Check sheet for the modelled part. Datum: model origin and axes. Units: mm. Face numbers are marked on the shaded views. A direction names the side the tool comes from. Give positions to 0.01 mm unless a question says otherwise; leave off trailing zeros. Write each loop counter-clockwise with the first axis right and the second up, starting at its lowest first coordinate (ties: lowest second). Pieces come first, ordered by that corner, then holes. Notation, with made-up numbers: M 17.5,-37 L 33.5,-37 A19 cw 33.5,-2 Z; hole C 3,17 d6. An arc over 180 degrees is marked long. Use CSV: the item, a comma, the result in double quotes. Start each with the question number.
1. Depth check by flat-ended pin: P1, Ø0.6, axis at y = 0, z = 0.5, coming from the -X side; P2, Ø1, axis at x = -1.5, y = -1, coming from the -Z side. Enter the tip coordinate at first touch or a pass-through.
2. Access from +Z, -Z, +X, -X, +Y, -Y to the whole of each face (thin tool, end or side, straight path). Record for the marked faces 5, 6, 7, 8 and 9.
3. Mould release check, pull along X, two halves, no side actions. Record for the marked faces 1, 2, 3 and 4: +X half, -X half, draft (parallel to the pull), parting line (faces both ways), or undercut.
4. Cross-section at A-A, the plane z = 1.4. Enter the section's corners in (x, y) (3 decimals), and give its area (3 significant figures).
5. Scan lines: line 1 (X direction, y = 1.5, z = 1.35); line 2 (Z direction, x = -3, y = 1); line 3 (Z direction, x = -1.25, y = 1.5). Record each from-to range of solid material in increasing order.
6. Cross-section at D-D, the plane z = 2.5. Enter the section's corners in (x, y).
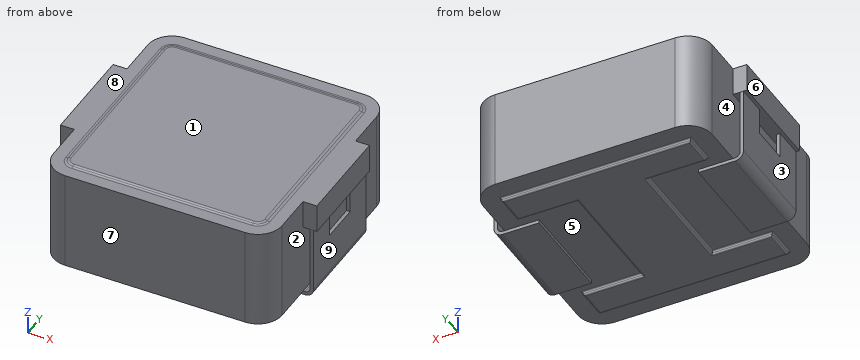
from build123d import *

# Parameters (mm, degrees)
SKETCH1_W            = 6.6
SKETCH1_H            = 6.6
BOSS_EXTRUDE1_DEPTH  = 2.9
SKETCH6_W            = 7.4
SKETCH6_H            = 2.9
BOSS_EXTRUDE5_DEPTH  = 0.85
FILLET1_R            = 0.7
SKETCH2_W            = 0.9
SKETCH2_H            = 2.1
CUT_EXTRUDE1_DEPTH   = 0.05
SKETCH3_W            = 1.3
SKETCH3_H            = 2.89
BOSS_EXTRUDE2_DEPTH  = 0.15
SKETCH4_W            = 0.3
SKETCH4_H            = 2.89
BOSS_EXTRUDE3_DEPTH  = 2
FILLET2_R            = 0.25
BOSS_EXTRUDE4_DEPTH  = 0.1
FILLET3_R            = 0.05
FILLET4_R            = 0.05
SKETCH8_W            = 0.2
SKETCH8_H            = 2.89
CUT_EXTRUDE2_DEPTH   = 2.05
FILLET5_R            = 0.15
SKETCH9_W            = 0.75
SKETCH9_H            = 1.15
CUT_EXTRUDE3_DEPTH   = 0.1
FILLET2_OF_MIRROR2_R = 0.25
FILLET5_OF_MIRROR2_R = 0.15
SKETCH10_W           = 10
SKETCH10_H           = 10
CUT_EXTRUDE4_DEPTH   = 0.03
FILLET6_R            = 0.2
FILLET7_R            = 0.2


# Some blends are built 0.0001 mm under size
with BuildPart() as part:
    # Sketch1 → Boss-Extrude1 (new body)
    with BuildSketch(Plane.XY):
        Rectangle(SKETCH1_W, SKETCH1_H)
    extrude(amount=BOSS_EXTRUDE1_DEPTH)

    # Sketch6 → Boss-Extrude5 (add)
    with BuildSketch(Plane.XY.offset(2.9)):
        Rectangle(SKETCH6_W, SKETCH6_H)
    extrude(amount=-BOSS_EXTRUDE5_DEPTH)

    # Fillet1
    fillet1_edges = [part.edges().sort_by_distance(p)[0] for p in [
        (3.3, -3.3, 1.45),
        (-3.3, -3.3, 1.45),
        (-3.3, 3.3, 1.45),
        (3.3, 3.3, 1.45),
    ]]
    fillet(fillet1_edges, radius=FILLET1_R)

    # Sketch2 → Cut-Extrude1 (cut)
    with BuildSketch(Plane(origin=(0, 0, 0), x_dir=(-1, 0, 0), z_dir=(0, 0, -1))):
        with Locations((2.85, 0)):
            Rectangle(SKETCH2_W, SKETCH2_H)
        with Locations((-2.85, 0)):
            Rectangle(SKETCH2_W, SKETCH2_H)
    extrude(amount=-CUT_EXTRUDE1_DEPTH, mode=Mode.SUBTRACT)

    # Sketch3 → Boss-Extrude2 (add)
    with BuildSketch(Plane(origin=(0, 0, 0.05), x_dir=(-1, 0, 0), z_dir=(0, 0, -1))):
        with Locations((2.95, 0)):
            Rectangle(SKETCH3_W, SKETCH3_H)
    boss_extrude2 = extrude(amount=BOSS_EXTRUDE2_DEPTH)

    # Sketch4 → Boss-Extrude3 (add)
    with BuildSketch(Plane.XY.offset(0.05)):
        with Locations((-3.45, 0)):
            Rectangle(SKETCH4_W, SKETCH4_H)
    boss_extrude3 = extrude(amount=BOSS_EXTRUDE3_DEPTH)

    # Fillet2
    fillet2_edges = [part.edges().sort_by_distance(p)[0] for p in [
        (-3.6, 0, -0.1),
    ]]
    fillet(fillet2_edges, radius=FILLET2_R)

    # Sketch5 → Boss-Extrude4 (add)
    with BuildSketch(Plane(origin=(0, 0, 0), x_dir=(-1, 0, 0), z_dir=(0, 0, -1))):
        Polygon((2.725, -2.7), (-2.725, -2.7), (-2.725, -1.8), (-1, -1.8), (-1, 1.8), (-2.725, 1.8), (-2.725, 2.7), (2.725, 2.7), (2.725, 1.8), (1, 1.8), (1, -1.8), (2.725, -1.8), align=None)
    extrude(amount=BOSS_EXTRUDE4_DEPTH)

    # Fillet3
    fillet3_edges = [part.edges().sort_by_distance(p)[0] for p in [
        (-2.725, -2.25, -0.1),
        (-1.8625, -1.8, -0.1),
        (-1, 0, -0.1),
        (-1.8625, 1.8, -0.1),
        (-2.725, 2.25, -0.1),
        (0, 2.7, -0.1),
        (2.725, 2.25, -0.1),
        (1.8625, 1.8, -0.1),
        (1, 0, -0.1),
        (1.8625, -1.8, -0.1),
        (2.725, -2.25, -0.1),
        (0, -2.7, -0.1),
    ]]
    fillet(fillet3_edges, radius=FILLET3_R)

    # Fillet4
    fillet4_edges = [part.edges().sort_by_distance(p)[0] for p in [
        (-1.8625, 1.8, 0),
        (-2.725, 2.25, 0),
        (0, 2.7, 0),
        (2.725, 2.25, 0),
        (1.8625, 1.8, 0),
        (1, 0, 0),
        (1.8625, -1.8, 0),
        (2.725, -2.25, 0),
        (0, -2.7, 0),
        (-1, 0, 0),
        (-2.725, -2.25, 0),
        (-1.8625, -1.8, 0),
    ]]
    fillet(fillet4_edges, radius=FILLET4_R - 0.0001)  # a hair under: the kernel refuses the full size

    # Sketch8 → Cut-Extrude2 (cut)
    with BuildSketch(Plane(origin=(0, 0, 0), x_dir=(-1, 0, 0), z_dir=(0, 0, -1))):
        with Locations((3.4, 0)):
            Rectangle(SKETCH8_W, SKETCH8_H)
    cut_extrude2 = extrude(amount=-CUT_EXTRUDE2_DEPTH, mode=Mode.SUBTRACT)

    # Fillet5
    fillet5_edges = [part.edges().sort_by_distance(p)[0] for p in [
        (-3.5, 0, 0),
    ]]
    fillet(fillet5_edges, radius=FILLET5_R)

    # Sketch9 → Cut-Extrude3 (cut)
    with BuildSketch(Plane.ZY.offset(3.6)):
        with Locations((1.675, 0)):
            Rectangle(SKETCH9_W, SKETCH9_H)
    cut_extrude3 = extrude(amount=-CUT_EXTRUDE3_DEPTH, mode=Mode.SUBTRACT)

    # Mirror2: Boss-Extrude2, Boss-Extrude3, Cut-Extrude2, Cut-Extrude3 across plane
    add(boss_extrude2.mirror(Plane(origin=(0, 0, 0), x_dir=(0, 0, 1), z_dir=(1, 0, 0))))
    add(boss_extrude3.mirror(Plane(origin=(0, 0, 0), x_dir=(0, 0, 1), z_dir=(1, 0, 0))))
    add(cut_extrude2.mirror(Plane(origin=(0, 0, 0), x_dir=(0, 0, 1), z_dir=(1, 0, 0))), mode=Mode.SUBTRACT)
    add(cut_extrude3.mirror(Plane(origin=(0, 0, 0), x_dir=(0, 0, 1), z_dir=(1, 0, 0))), mode=Mode.SUBTRACT)

    # Fillet2 of Mirror2
    fillet2_of_mirror2_edges = [part.edges().sort_by_distance(p)[0] for p in [
        (3.6, 0, -0.1),
    ]]
    fillet(fillet2_of_mirror2_edges, radius=FILLET2_OF_MIRROR2_R)

    # Fillet5 of Mirror2
    fillet5_of_mirror2_edges = [part.edges().sort_by_distance(p)[0] for p in [
        (3.5, 0, 0),
    ]]
    fillet(fillet5_of_mirror2_edges, radius=FILLET5_OF_MIRROR2_R)

    # Sketch10 → Cut-Extrude4 (cut)
    with BuildSketch(Plane.XY.offset(2.9)):
        with Locations((0.5029938, 0.413168945)):
            Rectangle(SKETCH10_W, SKETCH10_H)
        with BuildLine():
            Line((-2.6, 2.9), (2.6, 2.9))
            ThreePointArc((2.6, 2.9), (2.812132034, 2.812132034), (2.9, 2.6))
            Line((2.9, 2.6), (2.9, -2.6))
            ThreePointArc((2.9, -2.6), (2.812132034, -2.812132034), (2.6, -2.9))
            Line((2.6, -2.9), (-2.6, -2.9))
            ThreePointArc((-2.6, -2.9), (-2.812132034, -2.812132034), (-2.9, -2.6))
            Line((-2.9, -2.6), (-2.9, 2.6))
            ThreePointArc((-2.9, 2.6), (-2.812132034, 2.812132034), (-2.6, 2.9))
        make_face(mode=Mode.SUBTRACT)
    extrude(amount=-CUT_EXTRUDE4_DEPTH, mode=Mode.SUBTRACT)

    # Fillet6
    # the kernel refuses this fillet: 0.2 mm, written as the material it takes off along each edge
    with BuildSketch(Plane(origin=(-2.6, -2.6, 2.9), x_dir=(0, -1, 0), z_dir=(1, 0, 0))) as fillet6_piece_1:
        with BuildLine():
            CenterArc((0.194643462, 0.2), FILLET6_R, 270, 31.788330618)
            Line((0.194643462, 0), (0.194643462, -0.004))
            Line((0.194643462, -0.004), (0.3, -0.004))
            Line((0.3, -0.004), (0.304, 0))
            ThreePointArc((0.304, 0), (0.304, 0.015), (0.302107131, 0.0266))
            Line((0.302107131, 0.0266), (0.3, 0.03))
        make_face()
    revolve(axis=Axis((-2.6, -2.6, 2.9), (0, 0, -1)), revolution_arc=90, mode=Mode.SUBTRACT)
    with BuildSketch(Plane(origin=(-2.9, -2.6, 2.9), x_dir=(1.837049031358635e-11, 0, -1.0), z_dir=(0, 1, 0)), Plane(origin=(-2.6, 2.9, 2.9), x_dir=(0, -1.837049031358635e-11, -1.0), z_dir=(1, 0, 0)), Plane(origin=(2.9, 2.6, 2.9), x_dir=(-1.837049031358635e-11, 0, -1.0), z_dir=(0, -1, 0)), Plane(origin=(2.6, -2.9, 2.9), x_dir=(0, 1.837049031358635e-11, -1.0), z_dir=(-1, 0, 0))) as fillet6_piece_2:
        with BuildLine():
            CenterArc((0.2, -0.105356538), FILLET6_R, 148.211669384, 31.788330618)
            Line((0, -0.105356538), (-0.004, -0.105356538))
            Line((-0.004, -0.105356538), (-0.004, 0))
            Line((-0.004, 0), (0, 0.004))
            ThreePointArc((0, 0.004), (0.015, 0.004), (0.0266, 0.002107131))
            Line((0.0266, 0.002107131), (0.03, 0))
        make_face()
    extrude(amount=5.2, mode=Mode.SUBTRACT)
    with BuildSketch(Plane(origin=(-2.6, 2.6, 2.9), x_dir=(-1, 0, 0), z_dir=(0, -1, 0))) as fillet6_piece_3:
        with BuildLine():
            CenterArc((0.194643462, 0.2), FILLET6_R, 270, 31.788330618)
            Line((0.194643462, 0), (0.194643462, -0.004))
            Line((0.194643462, -0.004), (0.3, -0.004))
            Line((0.3, -0.004), (0.304, 0))
            ThreePointArc((0.304, 0), (0.304, 0.015), (0.302107131, 0.0266))
            Line((0.302107131, 0.0266), (0.3, 0.03))
        make_face()
    revolve(axis=Axis((-2.6, 2.6, 2.9), (0, 0, -1)), revolution_arc=90, mode=Mode.SUBTRACT)
    with BuildSketch(Plane(origin=(2.6, 2.6, 2.9), x_dir=(0, 1, 0), z_dir=(-1, 0, 0))) as fillet6_piece_4:
        with BuildLine():
            CenterArc((0.194643462, 0.2), FILLET6_R, 270, 31.788330618)
            Line((0.194643462, 0), (0.194643462, -0.004))
            Line((0.194643462, -0.004), (0.3, -0.004))
            Line((0.3, -0.004), (0.304, 0))
            ThreePointArc((0.304, 0), (0.304, 0.015), (0.302107131, 0.0266))
            Line((0.302107131, 0.0266), (0.3, 0.03))
        make_face()
    revolve(axis=Axis((2.6, 2.6, 2.9), (0, 0, -1)), revolution_arc=90, mode=Mode.SUBTRACT)
    with BuildSketch(Plane(origin=(2.6, -2.6, 2.9), x_dir=(1, 0, 0), z_dir=(0, 1, 0))) as fillet6_piece_5:
        with BuildLine():
            CenterArc((0.194643462, 0.2), FILLET6_R, 270, 31.788330618)
            Line((0.194643462, 0), (0.194643462, -0.004))
            Line((0.194643462, -0.004), (0.3, -0.004))
            Line((0.3, -0.004), (0.304, 0))
            ThreePointArc((0.304, 0), (0.304, 0.015), (0.302107131, 0.0266))
            Line((0.302107131, 0.0266), (0.3, 0.03))
        make_face()
    revolve(axis=Axis((2.6, -2.6, 2.9), (0, 0, -1)), revolution_arc=90, mode=Mode.SUBTRACT)

    # Fillet7
    fillet7_edges = [part.edges().sort_by_distance(p)[0] for p in [
        (0, 2.9, 2.87),
        (-2.812132034, 2.812132034, 2.87),
        (-2.9, 0, 2.87),
        (-2.812132034, -2.812132034, 2.87),
        (0, -2.9, 2.87),
        (2.812132034, -2.812132034, 2.87),
        (2.9, 0, 2.87),
        (2.812132034, 2.812132034, 2.87),
    ]]
    fillet(fillet7_edges, radius=FILLET7_R)


solid = part.part
Worked answers:
1,P1,"stops at x = -3.6"
1,P2,"stops at z = -0.05"
2,face 5,"-Z"
2,face 6,"+Z, -Z, -X, +Y, -Y"
2,face 7,"+Z, -Z, +X, -X, -Y"
2,face 8,"+Z"
2,face 9,"-Z, +X, +Y, -Y"
3,face 1,"draft"
3,face 2,"undercut"
3,face 3,"-X half"
3,face 4,"undercut"
4,outline,"M -3.6,-1.445 L -3.5,-1.445 L -3.5,-0.575 L -3.6,-0.575 Z; M -3.6,0.575 L -3.5,0.575 L -3.5,1.445 L -3.6,1.445 Z; M -3.3,-2.6 A0.7 ccw -2.6,-3.3 L 2.6,-3.3 A0.7 ccw 3.3,-2.6 L 3.3,2.6 A0.7 ccw 2.6,3.3 L -2.6,3.3 A0.7 ccw -3.3,2.6 Z; M 3.5,-1.445 L 3.6,-1.445 L 3.6,-0.575 L 3.5,-0.575 Z; M 3.5,0.575 L 3.6,0.575 L 3.6,1.445 L 3.5,1.445 Z"
4,area,"43.5 mm^2"
5,line 1,"x = -3.3 to 3.3"
5,line 2,"z = -0.1 to 2.87"
5,line 3,"z = 0 to 2.9"
6,outline,"M -3.7,-1.45 L -3.3,-1.45 L -3.3,-2.6 A0.7 ccw -2.6,-3.3 L 2.6,-3.3 A0.7 ccw 3.3,-2.6 L 3.3,-1.45 L 3.7,-1.45 L 3.7,1.45 L 3.3,1.45 L 3.3,2.6 A0.7 ccw 2.6,3.3 L -2.6,3.3 A0.7 ccw -3.3,2.6 L -3.3,1.45 L -3.7,1.45 Z"
